```python
from build123d import *

# Parameters (mm, degrees)
SKETCH1_W                      = 34.925
SKETCH1_H                      = 1.5875
F_1_16_0_0625_DIAMETER_HOLE1_D = 1.5875
CIRPATTERN1_COUNT              = 12


with BuildPart() as part:
    # Sketch1 → Revolve1 (revolve)
    with BuildSketch(Plane.XY):
        with Locations((-26.9875, 0.79375)):
            Rectangle(SKETCH1_W, SKETCH1_H)
    revolve(axis=Axis((0, 55, 0), (0, -1, 0)))

    # 1/16 (0.0625) Diameter Hole1 (through all)
    with Locations(Plane(origin=(0, 1.5875, 0), x_dir=(1, 0, 0), z_dir=(0, 1, 0))):
        with Locations((-41.275, 0)):
            f_1_16_0_0625_diameter_hole1 = Hole(F_1_16_0_0625_DIAMETER_HOLE1_D / 2)

    # CirPattern1: 1/16 (0.0625) Diameter Hole1 ×12 about axis
    cirpattern1_axis = Axis((0, 0, 0), (0, 1, 0))
    for i in range(1, CIRPATTERN1_COUNT):
        add(f_1_16_0_0625_diameter_hole1.rotate(cirpattern1_axis, i * 360 / CIRPATTERN1_COUNT), mode=Mode.SUBTRACT)


solid = part.part
```
Part model, mm, in its own coordinate system. Give positions to 0.01 mm unless a question says otherwise; leave off trailing zeros. Loops run counter-clockwise (first coordinate to the right, second up) from the corner with the lowest first, then second, coordinate; pieces in that order, holes last. Notation, with made-up numbers: M -17.5,20 L -0.5,20 A20 ccw -0.5,34 Z; hole C 35.5,51 d7. An arc over 180 degrees is marked long. Return JSON: item names as keys, results as strings.
1) Pull direction Z, two halves, no side cores. Call faces 1 (the face through (-4.4, 0.8, 8.45)), 2 (the face through (11, 0, -1)), 3 (the face through (-42.397, 0.805, -13.352)): released by +Z, released by -Z, zero draft, split by the parting line, or undercut.
Calculated:
{"face 1": "undercut", "face 2": "zero draft", "face 3": "split by the parting line"}
2) Saw through at C-C, the plane z = -31. List the corners of the cut face in (x, y).
Calculated:
{"outline": "M -31.86,0 L 31.86,0 L 31.86,1.59 L -31.86,1.59 Z"}
3) Drill centre lines: line 1 (X direction, y = 1.15, z = 2.5); line 2 (Z direction, x = 4.5, y = 0.9); line 3 (Z direction, x = 1.5, y = 0.8). Where is each one in solid material? Low to high.
Calculated:
{"line 1": "x = -44.38 to -9.19, 9.19 to 44.38", "line 2": "z = -44.22 to -8.39, 8.39 to 44.22", "line 3": "z = -44.42 to -9.41, 9.41 to 44.42"}
4) Saw through at B-B, the plane x = -22.5. List the corners of the cut face in (y, z), then the cut area to 3 significant figures.
Calculated:
{"outline": "M 0,-38.33 L 1.59,-38.33 L 1.59,38.33 L 0,38.33 Z", "area": "122 mm2"}
5) Saw through at A-A, the plane y = 0.6. Count the separate pieces of the cut face and the enclosed holes in it, then the cut area to 3 significant figures.
Calculated:
{"separate pieces": "1", "enclosed holes": "13", "area": "5,900 mm2"}
